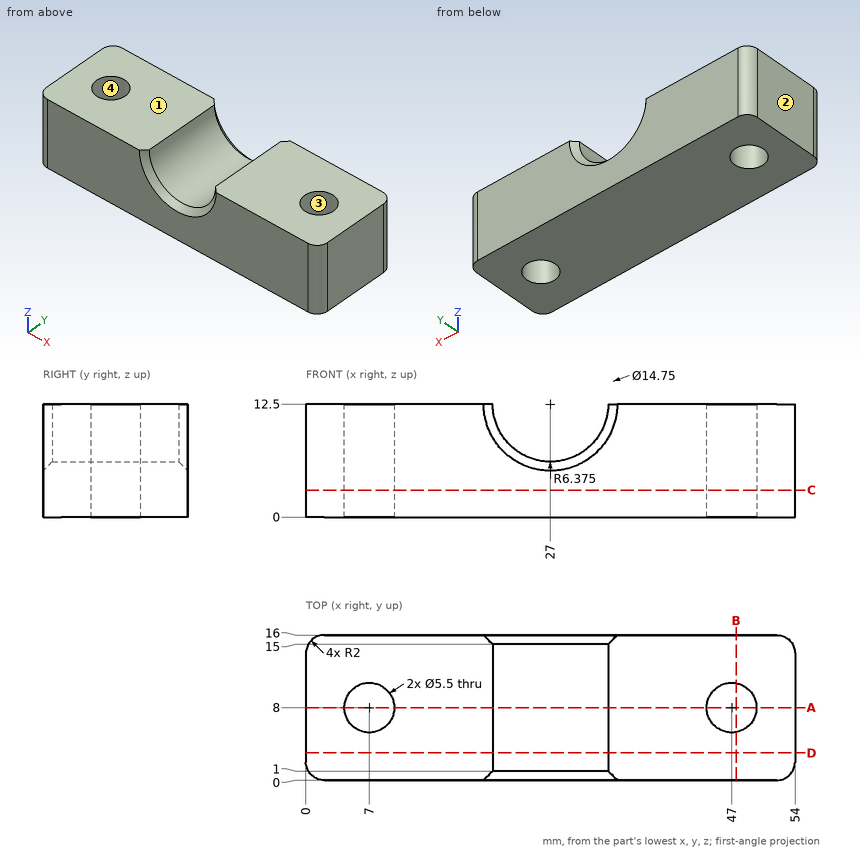
Verification items for this drawing (mm, ordinates from the low corner). Coordinates: 2 decimals unless noted, no trailing zeros. Order: outer loops, then holes, each group sorted by start corner. A loop starts at its lowest first (then second) coordinate and runs counter-clockwise, first axis right, second up. Notation, with made-up numbers: (-15.75, 30.5) - (29.25, 30.5) arc R18 cw to (29.25, 54.5) - close; hole circle Ø3 at (84.5, 67). An arc over 180 degrees is marked (long way). Answer as a JSON object with one key per item and string values. Group by question number.
Item 1: Draft check along X on the marked faces 1, 2, 3 and 4. Enter one of: +X half, -X half, draft (parallel to the pull), parting line (faces both ways), or undercut.
Item 2: Sectioned sample at D-D, the plane y = 3. Record the cut outline in (x, z) (3 decimals), and give its area (3 significant figures).
Item 3: Depth check by flat-ended pin: pin 1 Ø7 at (x, y) = (47, 8) entering from +Z. Enter the tip coordinate at first touch or a pass-through.
Item 4: Sectioned sample at B-B, the plane x = 47.5. Record the cut outline in (y, z).
Item 5: Sectioned sample at A-A, the plane y = 8. Record the cut outline in (x, z) (3 decimals).
Item 6: Sectioned sample at C-C, the plane z = 3. Record the cut outline in (x, y), and give its area (3 significant figures).
Item 7: Scan lines: probe 1 along Y at (x, z) = (7, 3.25); probe 2 along X at (y, z) = (7.5, 8.75); probe 3 along X at (y, z) = (10.5, 8). Record each from-to range of solid material in increasing order.
Resolved:
{
 "1": {"face 1": "draft", "face 2": "-X half", "face 3": "undercut", "face 4": "undercut"},
 "2": {"outline": "(0, 0) - (54, 0) - (54, 12.5) - (33.375, 12.5) arc R6.375 cw to (20.625, 12.5) - (0, 12.5) - close", "area": "611 mm^2"},
 "3": {"pin 1": "z = 12.5"},
 "4": {"outline": "(0, 0) - (5.3, 0) - (5.3, 12.5) - (0, 12.5) - close; (10.7, 0) - (16, 0) - (16, 12.5) - (10.7, 12.5) - close"},
 "5": {"outline": "(0, 0) - (4.25, 0) - (4.25, 12.5) - (0, 12.5) - close; (9.75, 0) - (44.25, 0) - (44.25, 12.5) - (33.375, 12.5) arc R6.375 cw to (20.625, 12.5) - (9.75, 12.5) - close; (49.75, 0) - (54, 0) - (54, 12.5) - (49.75, 12.5) - close"},
 "6": {"outline": "(0, 2) arc R2 ccw to (2, 0) - (52, 0) arc R2 ccw to (54, 2) - (54, 14) arc R2 ccw to (52, 16) - (2, 16) arc R2 ccw to (0, 14) - close; hole circle Ø5.5 at (7, 8); hole circle Ø5.5 at (47, 8)", "area": "813 mm^2"},
 "7": {"probe 1": "0 to 5.25, 10.75 to 16", "probe 2": "0 to 4.3, 9.7 to 21.84, 32.16 to 44.3, 49.7 to 54", "probe 3": "0 to 5.85, 8.15 to 22.48, 31.52 to 45.85, 48.15 to 54"}
}
